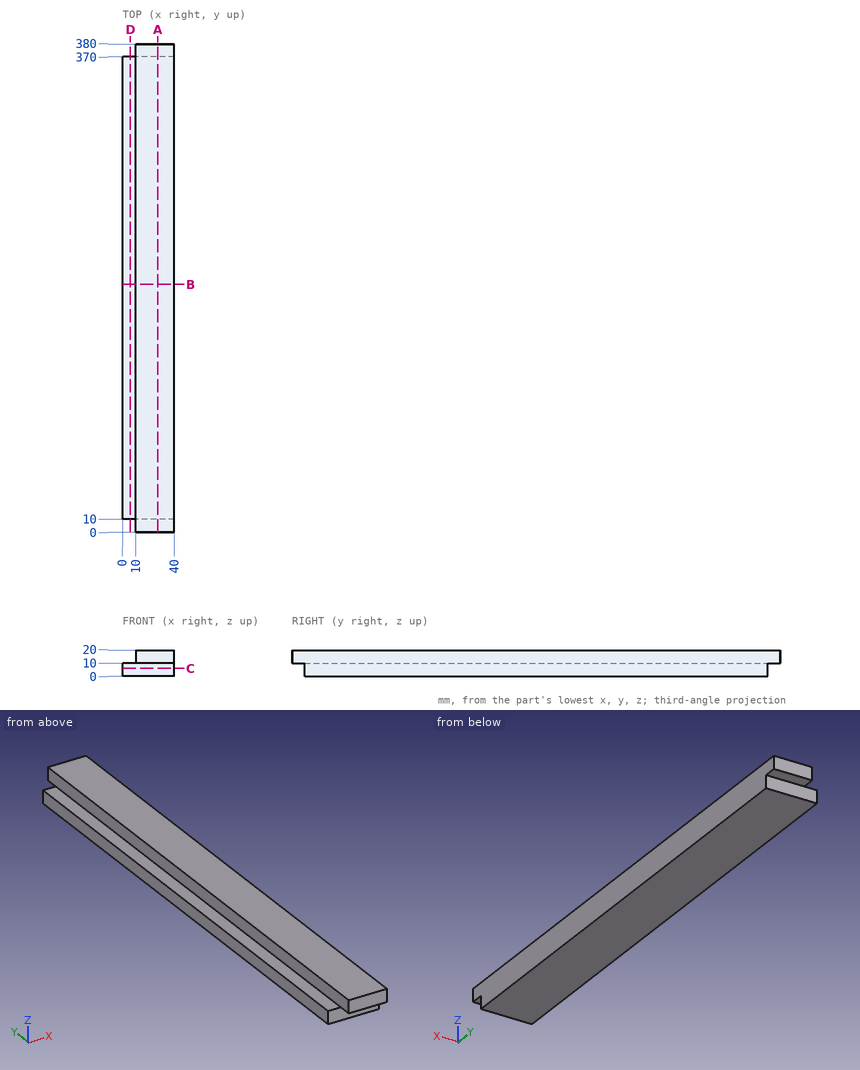
Job drawing, mm, ordinate dimensions from the low corner. One solid piece. Give positions to 0.01 mm unless a question says otherwise; leave off trailing zeros. Order: outer loops, then holes, each group sorted by start corner. A loop starts at its lowest first (then second) coordinate and runs counter-clockwise, first axis right, second up. Notation, with made-up numbers: (17, -13) - (26, -13) arc R30 ccw to (26, 11) - close; hole circle Ø10 at (57.5, 77). An arc over 180 degrees is marked (long way). Return JSON: item names as keys, results as strings.
1) Flat gauge pins, fed straight in: P1, Ø4, axis at x = 5, z = 10, coming from the -Y side; P2, Ø6, axis at x = 15.5, z = 5.5, coming from the +Y side; P3, Ø8, axis at y = 195, z = 16, coming from the -X side. Where does each tip first touch, or does it go through?
Geometry says:
{"P1": "y = 10", "P2": "y = 370", "P3": "x = 10"}
2) Cut at A-A, the plane x = 27.5. Give the cut face in (y, z), plus the area to 3 significant figures.
Geometry says:
{"outline": "(0, 10) - (10, 10) - (10, 0) - (370, 0) - (370, 10) - (380, 10) - (380, 20) - (0, 20) - close", "area": "7,400 mm²"}
3) Probe line 1 (Y direction, x = 36.5, z = 9.25); line 2 (Z direction, x = 7, y = 91); line 3 (X direction, y = 270.5, z = 12.5). List the from-to ranges inside material, lowest first. Write a range as from..to.
Geometry says:
{"line 1": "10..370", "line 2": "0..10", "line 3": "10..40"}
4) Cut at C-C, the plane z = 6. Give the cut face in (x, y).
Geometry says:
{"outline": "(0, 10) - (40, 10) - (40, 370) - (0, 370) - close"}
5) Cut at D-D, the plane x = 6. Give the cut face in (y, z).
Geometry says:
{"outline": "(10, 0) - (370, 0) - (370, 10) - (10, 10) - close"}
6) Cut at B-B, the plane y = 193. Give the cut face in (x, z).
Geometry says:
{"outline": "(0, 0) - (40, 0) - (40, 20) - (10, 20) - (10, 10) - (0, 10) - close"}
